```python
from build123d import *

# Parameters (mm, degrees)
BOSS_EXTRUDE1_DEPTH = 11.1125
SKETCH2_R           = 3.5687
CUT_EXTRUDE1_DEPTH  = 26.4
SKETCH3_R           = 3.5687
CUT_EXTRUDE2_DEPTH  = 26.4


with BuildPart() as part:
    # Sketch1 → Boss-Extrude1 (new body, symmetric)
    with BuildSketch(Plane.XY):
        with BuildLine():
            Line((0, 0), (0, 25.4))
            ThreePointArc((0, 25.4), (3.376576302, 24.001376302), (4.7752, 20.6248))
            Line((4.7752, 20.6248), (4.7752, 7.9502))
            ThreePointArc((4.7752, 7.9502), (5.70513597, 5.70513597), (7.9502, 4.7752))
            Line((7.9502, 4.7752), (20.6248, 4.7752))
            ThreePointArc((20.6248, 4.7752), (24.001376302, 3.376576302), (25.4, 0))
            Line((25.4, 0), (0, 0))
        make_face()
    extrude(amount=BOSS_EXTRUDE1_DEPTH, both=True)

    # Sketch2 → Cut-Extrude1 (cut, through all)
    with BuildSketch(Plane(origin=(0, 0, 0), x_dir=(1, 0, 0), z_dir=(0, 1, 0))):
        with Locations((12.7, 0)):
            Circle(SKETCH2_R)
    extrude(amount=CUT_EXTRUDE1_DEPTH, mode=Mode.SUBTRACT)

    # Sketch3 → Cut-Extrude2 (cut, through all)
    with BuildSketch(Plane(origin=(0, 0, 0), x_dir=(0, 0, -1), z_dir=(1, 0, 0))):
        with Locations((0, 12.7)):
            Circle(SKETCH3_R)
    extrude(amount=CUT_EXTRUDE2_DEPTH, mode=Mode.SUBTRACT)


solid = part.part
```
For this review, take the finished solid that the model builds, in its own axes (mm). A direction names the side the tool comes from. Give positions to 0.01 mm unless a question says otherwise; leave off trailing zeros. Loops run counter-clockwise (first coordinate to the right, second up) from the corner with the lowest first, then second, coordinate; pieces in that order, holes last. Notation, with made-up numbers: M 28,73 L 68,73 A15 ccw 68,100 Z; hole C 6,46 d10. An arc over 180 degrees is marked long. One line per item, written item: value. Start each with the question number.
Q1. Draft analysis for pull direction Y (two halves, no side actions). For faces 1 (the face through (16, 0, 3)), 2 (the face through (3.34, 24.04, 0.16)), 3 (the face through (2.354, 9.216, 0.774)), 4 (the face through (7, 4, -11.112)), state which applies: released by +Y, released by -Y, zero draft, split by the parting line, or undercut.
Q2. Add section B-B (z = 0). Give the boundary of the cut face in (x, y) (3 decimals).
Q3. Machinability: for faces 5 (the face through (4.775, 17, 0)), 6 (the face through (0, 10, 3)), which of the approach directions +Z, -Z, +X, -X, +Y, -Y give a long, thin tool a straight path to every point of the face, cutting with its end or side? Answer none if there is none.
Q4. Clearance check with flat-ended pins moving along their axes: pin 1 Ø3 at (x, z) = (16, 7.5) entering from +Y; pin 2 Ø2 at (y, z) = (11.5, -8.5) entering from +X. State where each tip first meets the part, or that it passes through.
Q5. Add section D-D (z = -9). Give the boundary of the cut face in (x, y) (3 decimals), and give its area (3 significant figures).
Q6. For L1, parallel to Z at x = 12.7, y = 1; L2, parallel to Y at x = 20.75, z = 6.5; L3, parallel to X at y = 9, z = 5, list the stretches that pass through material, from the lowest coordinate up.
Q7. Add section A-A (y = 12.7). Give the boundary of the cut face in (x, z).
Reply:
1. face 1: released by -Y
1. face 2: released by +Y
1. face 3: undercut
1. face 4: zero draft
2. outline: M 0,0 L 9.131,0 L 9.131,4.775 L 7.95,4.775 A3.175 cw 4.775,7.95 L 4.775,9.131 L 0,9.131 Z; M 0,16.269 L 4.775,16.269 L 4.775,20.625 A4.775 ccw 0,25.4 Z; M 16.269,0 L 25.4,0 A4.775 ccw 20.625,4.775 L 16.269,4.775 Z
3. face 5: +Z, -Z, +X, +Y
3. face 6: +Z, -Z, -X, +Y, -Y
4. pin 1: y = 4.78
4. pin 2: x = 4.78
5. outline: M 0,0 L 25.4,0 A4.775 ccw 20.625,4.775 L 7.95,4.775 A3.175 cw 4.775,7.95 L 4.775,20.625 A4.775 ccw 0,25.4 Z
5. area: 212 mm²
6. L1: -11.11 to -3.57, 3.57 to 11.11
6. L2: 0 to 4.77
6. L3: 0 to 4.78
7. outline: M 0,-11.11 L 4.78,-11.11 L 4.78,-3.57 L 0,-3.57 Z; M 0,3.57 L 4.78,3.57 L 4.78,11.11 L 0,11.11 Z
